Autodesk Inventor part; units mm, degrees
ref_plane "YZ Plane" through (0, 0, 0) normal (1, 0, 0) x (0, 1, 0)
ref_plane "XZ Plane" through (0, 0, 0) normal (0, 1, 0) x (-1, 0, 0)
ref_plane "XY Plane" through (0, 0, 0) normal (0, 0, 1) x (1, 0, 0)
sketch "스케치1" plane through (0, 0, 0) normal (0, 1, 0) x (-1, 0, 0)
  line L0 (-10.9012, 33.5504) -> (10.9012, 33.5504)
  line L1 (10.9012, 33.5504) -> (28.5397, 20.7353)
  line L2 (28.5397, 20.7353) -> (35.277, 0)
  line L3 (35.277, 0) -> (28.5397, -20.7353)
  line L4 (28.5397, -20.7353) -> (10.9012, -33.5504)
  line L5 (10.9012, -33.5504) -> (-10.9012, -33.5504)
  line L6 (-10.9012, -33.5504) -> (-28.5397, -20.7353)
  line L7 (-28.5397, -20.7353) -> (-35.277, 0)
  line L8 (-35.277, 0) -> (-28.5397, 20.7353)
  line L9 (-28.5397, 20.7353) -> (-10.9012, 33.5504)
  line L10 (11.9409, -36.7504) -> (-11.9409, -36.7504)
  line L11 (-11.9409, -36.7504) -> (-31.2618, -22.713)
  line L12 (-31.2618, -22.713) -> (-38.6417, 0)
  line L13 (-38.6417, 0) -> (-31.2618, 22.713)
  line L14 (-31.2618, 22.713) -> (-11.9409, 36.7504)
  line L15 (-11.9409, 36.7504) -> (11.9409, 36.7504)
  line L16 (11.9409, 36.7504) -> (31.2618, 22.713)
  line L17 (31.2618, 22.713) -> (38.6417, 0)
  line L18 (38.6417, 0) -> (31.2618, -22.713)
  line L19 (31.2618, -22.713) -> (11.9409, -36.7504)
  point P0 (0, 0)
  point P1 (0, 0)
  point P2 (0, 0)
  dimension "d0" = 70.554
  dimension "d1" = 3.2
extrude "돌출1" add sketch "스케치1" along normal blind 3.7 contours L0 L1 L2 L3 L4 L5 L6 L7 L8 L9 | L10 L11 L12 L13 L14 L15 L16 L17 L18 L19
sketch "스케치2" plane through (0, 3.7, 0) normal (0, 1, 0) x (1, 0, 0)
  line L0 (-11.4211, 35.1504) -> (11.4211, 35.1504)
  line L1 (11.4211, 35.1504) -> (29.9007, 21.7242)
  line L2 (29.9007, 21.7242) -> (36.9593, 0)
  line L3 (36.9593, 0) -> (29.9007, -21.7242)
  line L4 (29.9007, -21.7242) -> (11.4211, -35.1504)
  line L5 (11.4211, -35.1504) -> (-11.4211, -35.1504)
  line L6 (-11.4211, -35.1504) -> (-29.9007, -21.7242)
  line L7 (-29.9007, -21.7242) -> (-36.9593, 0)
  line L8 (-36.9593, 0) -> (-29.9007, 21.7242)
  line L9 (-29.9007, 21.7242) -> (-11.4211, 35.1504)
  line L10 (-31.2618, 22.713) -> (-38.6417, 0)
  point P0 (0, 0)
  point P1 (0, 0)
  dimension "d4" = 1.6
extrude "돌출2" cut sketch "스케치2" against normal blind 1.2
sketch "스케치3" plane through (0, 2.5, 0) normal (0, 1, 0) x (1, 0, 0)
  line L0 (-10.7712, 33.1504) -> (10.7712, 33.1504)
  line L1 (10.7712, 33.1504) -> (28.1994, 20.4881)
  line L2 (28.1994, 20.4881) -> (34.8564, 0)
  line L3 (34.8564, 0) -> (28.1994, -20.4881)
  line L4 (28.1994, -20.4881) -> (10.7712, -33.1504)
  line L5 (10.7712, -33.1504) -> (-10.7712, -33.1504)
  line L6 (-10.7712, -33.1504) -> (-28.1994, -20.4881)
  line L7 (-28.1994, -20.4881) -> (-34.8564, 0)
  line L8 (-34.8564, 0) -> (-28.1994, 20.4881)
  line L9 (-28.1994, 20.4881) -> (-10.7712, 33.1504)
  line L10 (-29.9007, 21.7242) -> (-11.4211, 35.1504)
  point P0 (0, 0)
  point P1 (0, 0)
  dimension "d7" = 2
extrude "돌출3" add sketch "스케치3" along normal blind 0.6
fillet "모깎기1" radius 1.2 20 edges at (0, 3.7, 36.7504) (0, 0, 36.7504) (-21.6014, 3.7, 29.7317) (-21.6014, 0, 29.7317) (-34.9517, 3.7, 11.3565) (-34.9517, 3.7, -11.3565) (-21.6014, 3.7, -29.7317) (0, 3.7, -36.7504) (21.6014, 3.7, -29.7317) (34.9517, 3.7, -11.3565) (34.9517, 3.7, 11.3565) (21.6014, 3.7, 29.7317) (21.6014, 0, -29.7317) (0, 0, -36.7504) (-21.6014, 0, -29.7317) (-34.9517, 0, -11.3565) (-34.9517, 0, 11.3565) (34.9517, 0, -11.3565) (34.9517, 0, 11.3565) (21.6014, 0, 29.7317)
sketch "스케치12" plane through (0, 0, 0) normal (0, -1, 0) x (1, 0, 0)
  circle A0 centre (0, 0) radius 12.7
  dimension "d53" = 25.4
extrude "돌출12" add sketch "스케치12" along normal blind 10.16
sketch "스케치13" plane through (0, -10.16, 0) normal (0, -1, 0) x (1, 0, 0)
  circle A0 centre (0, 0) radius 4.5
  line L0 (-2.5981, 4.5) -> (2.5981, 4.5)
  line L1 (2.5981, 4.5) -> (5.1962, 0)
  line L2 (5.1962, 0) -> (2.5981, -4.5)
  line L3 (2.5981, -4.5) -> (-2.5981, -4.5)
  line L4 (-2.5981, -4.5) -> (-5.1962, 0)
  line L5 (-5.1962, 0) -> (-2.5981, 4.5)
  point P0 (-3.8971, 2.25)
  point P1 (-3.8971, -2.25)
  point P2 (0, 4.5)
  point P3 (0, -4.5)
  point P4 (3.8971, -2.25)
  point P5 (3.8971, 2.25)
  dimension "d56" = 9
extrude "돌출13" cut sketch "스케치13" against normal blind 12
sketch "스케치14" plane through (0, 0, 0) normal (0, -1, 0) x (1, 0, 0)
  circle A0 centre (-23, 0) radius 9
  circle A1 centre (-11.5, -19.9186) radius 9
  circle A2 centre (11.5, -19.9186) radius 9
  circle A3 centre (23, 0) radius 9
  circle A4 centre (11.5, 19.9186) radius 9
  circle A5 centre (-11.5, 19.9186) radius 9
  point P0 (0, 0)
  dimension "d61" = 18
  dimension "d62" = 23
  dimension "d65" = 360
extrude "돌출14" cut sketch "스케치14" against normal up to surface (3.1 mm away)
sketch "스케치17" plane through (0, 1.84, 0) normal (0, -1, 0) x (1, 0, 0)
  line L0 (-2.5981, 4.5) -> (2.5981, 4.5)
  line L1 (-5.1962, 0) -> (-2.5981, 4.5)
  line L2 (-2.5981, -4.5) -> (-5.1962, 0)
  line L3 (2.5981, -4.5) -> (-2.5981, -4.5)
  line L4 (5.1962, 0) -> (2.5981, -4.5)
  line L5 (2.5981, 4.5) -> (5.1962, 0)
  line L6 (-2.0207, 3.5) -> (2.0207, 3.5)
  line L7 (2.0207, 3.5) -> (4.0415, 0)
  line L8 (4.0415, 0) -> (2.0207, -3.5)
  line L9 (2.0207, -3.5) -> (-2.0207, -3.5)
  line L10 (-2.0207, -3.5) -> (-4.0415, 0)
  line L11 (-4.0415, 0) -> (-2.0207, 3.5)
  point P0 (0, 0)
  point P1 (0, 0)
  dimension "d87" = 1
extrude "돌출15" add sketch "스케치17" along normal blind 8.5
fillet "모깎기2" radius 0.5 6 edges at (0, -10.16, 4.5) (-3.8971, -10.16, 2.25) (-3.8971, -10.16, -2.25) (3.8971, -10.16, 2.25) (3.8971, -10.16, -2.25) (0, -10.16, -4.5)
equation "\"d76\" = 55deg"
properties part number "OV-PAM_n_10_bottom"
Can you work these out from the model? Positions are in its coordinate system, mm. A direction names the side the tool comes from. Round coordinates to 2 decimals unless told otherwise and drop trailing zeros. Write each loop counter-clockwise with the first axis right and the second up, starting at its lowest first coordinate (ties: lowest second). Pieces come first, ordered by that corner, then holes. Notation, with made-up numbers: M 34,83.5 L 47,83.5 A25 cw 47,116.5 Z; hole C -30.5,10.25 d3. An arc over 180 degrees is marked long. Use CSV: the item, a comma, the result in double quotes.
(1) I'm going to push flat-ended pins straight in: pin 1 (1.2 mm diameter, centred on x = 0, y = -2.5, fed in from +Z); pin 2 (20.5 mm diameter, centred on x = 11.5, z = 19.92, fed in from -Y); pin 3 (12 mm diameter, centred on x = 3, z = -15, fed in from +Y); pin 4 (3 mm diameter, centred on y = -2, z = 15, fed in from -X). Where does each tip first touch, or does it pass through?
Check values:
pin 1,"z = 12.7"
pin 2,"y = 0"
pin 3,"y = 3.1"
pin 4,"through"
(2) On a 3-axis mill with a long thin cutter (end or side, diameter ignored), from which of +Z, -Z, +X, -X, +Y, -Y can I reach the whole of each face in a straight line? I mean faces 5 (the flat face through (19.36, 2.8, -26.91)), 6 (the cylindrical face through (-21.535, 3.339, 29.357)), 7 (the flat face through (0, -2, 3.5)). Say none if no direction works.
Check values:
face 5,"+Y"
face 6,"+Z, -X, +Y"
face 7,"-Y"
(3) Imagine slicing it at C-C (z = -1). Count the separate pieces of the cut face and the enclosed holes in it, plus the area to 3 significant figures.
Check values:
separate pieces,"3"
enclosed holes,"0"
area,"291 mm^2"
(4) Imagine slicing it at A-A (y = -1.5). Write out the boundary of the cut face in (x, z).
Check values:
outline,"C 0,0 d25.4; hole M -4.04,0 L -2.02,-3.5 L 2.02,-3.5 L 4.04,0 L 2.02,3.5 L -2.02,3.5 Z"
(5) We'd pull the mould along X, two halves only. Please class faces 1 (the flat face through (21.466, 1.841, -29.83)), 2 (the flat face through (3.045, -2.351, -1.726)), 3 (the flat face through (-35.003, 1.841, -11.198)), 4 (the flat face through (-3.915, -8.181, 2.218)): +X half, -X half, draft (parallel to the pull), parting line (faces both ways), or undercut.
Check values:
face 1,"+X half"
face 2,"undercut"
face 3,"-X half"
face 4,"undercut"
(6) I need wall thicknesses on line 1 along Z through (x, y) = (11.5, 1.5); line 2 along X through (y, z) = (2, 20.5); line 3 along X through (y, z) = (2.25, 3). Which ranges of each line are inside material? Lowest first, please.
Check values:
line 1,"-36.75 to -28.92, -10.92 to 10.92, 28.92 to 36.75"
line 2,"-31.98 to -20.48, -2.52 to 2.52, 20.48 to 31.98"
line 3,"-37.67 to -31.49, -14.51 to 14.51, 31.49 to 37.67"
